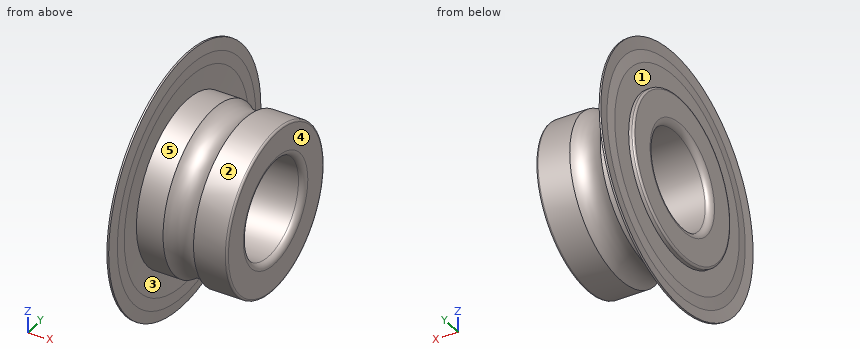
Autodesk Inventor part; units mm, degrees
ref_plane "YZ Plane" through (0, 0, 0) normal (1, 0, 0) x (0, 1, 0)
ref_plane "XZ Plane" through (0, 0, 0) normal (0, 1, 0) x (-1, 0, 0)
ref_plane "XY Plane" through (0, 0, 0) normal (0, 0, 1) x (1, 0, 0)
sketch "Sketch_62" plane through (0, 0, 0) normal (0, 0, 1) x (1, 0, 0)
  line L0 (50, 0) -> (-50, 0)
  line L1 (0, 4.1) -> (0, 2.8)
  arc A0 (0, 2.8) -> (0.3, 2.5) centre (0.3, 2.8) ccw
  line L2 (0.3, 2.5) -> (4.7, 2.5)
  arc A1 (4.7, 2.5) -> (5, 2.8) centre (4.7, 2.8) ccw
  line L3 (5, 2.8) -> (5, 4.1)
  arc A2 (5, 4.1) -> (4.9, 4.2) centre (4.9, 4.1) ccw
  line L4 (4.9, 4.2) -> (3.2793, 4.2)
  arc A3 (1.7207, 4.2) -> (3.2793, 4.2) centre (2.5, 5.1) ccw
  line L5 (1.7207, 4.2) -> (0.1, 4.2)
  arc A4 (0.1, 4.2) -> (0, 4.1) centre (0.1, 4.1) ccw
revolve "Revolution1" add sketch "Sketch_62" angle 360 about axis through (50, 0, 0) along (1, 0, 0)
sketch "Sketch_63" plane through (0, 0, 0) normal (0, 0, 1) x (1, 0, 0)
  line L0 (50, 0) -> (-50, 0)
  line L1 (0.27, 6.61) -> (0.315, 6.0075)
  line L2 (0.315, 6.0075) -> (0.27, 5.405)
  line L3 (0.27, 5.405) -> (0.27, 4.2)
  line L4 (0.27, 4.2) -> (0.36, 4.2)
  line L5 (0.36, 4.2) -> (0.45, 5.405)
  line L6 (0.45, 5.405) -> (0.45, 6.0075)
  line L7 (0.45, 6.0075) -> (0.36, 6.61)
  line L8 (0.36, 6.61) -> (0.27, 6.61)
revolve "Revolution2" add sketch "Sketch_63" angle 360 about axis through (50, 0, 0) along (1, 0, 0)
properties part number "625-Z_PART1"
For this review, take the finished solid that the model builds, in its own axes (mm). Face numbers are marked on the shaded views. A direction names the side the tool comes from. Round coordinates to 2 decimals unless told otherwise and drop trailing zeros. Loops run counter-clockwise (first coordinate to the right, second up) from the corner with the lowest first, then second, coordinate; pieces in that order, holes last. Notation, with made-up numbers: (-36.75, 46.5) - (20.25, 46.5) arc R14 cw to (20.25, 64.5) - close; hole circle Ø6 at (45, 21.5). An arc over 180 degrees is marked (long way). Put each result on its own line as item: value. Start each with the question number.
1. Mouldability with a two-part tool opening along Y and no side actions: class the marked faces 1, 2 and 3 as +Y half, -Y half, draft (parallel to the pull), parting line (faces both ways), or undercut.
2. For probe 1 along Z at (x, y) = (1.7, 0); probe 2 along Y at (x, z) = (3.6, 0.5); probe 3 along Z at (x, y) = (1.8, 0), list the stretches that pass through material, from the lowest coordinate up. Write a range as [from, to].
3. Consider section A-A on x = 4.5. State the section outline as (y, z) points.
4. For the marked faces 4 and 5, list the 3-axis set-ups (+Z, -Z, +X, -X, +Y, -Y) from which the entire face can be reached by the end or side of a thin tool; tool diameter is ignored.
5. Consider section B-B on x = 2.75. State the section outline as (y, z) points.
6. Insertion check: P1, Ø4, axis at y = -0.5, z = -0.5, coming from the -X side; P2, Ø2, axis at x = 3.5, z = -0.5, coming from the +Y side; P3, Ø1, axis at x = 1, z = 2, coming from the +Y side. Each pin has a flat end and moves straight along its axis. Give the tip position at first contact, or say it passes through.
Result sheet:
1. face 1: draft
1. face 2: parting line
1. face 3: undercut
2. probe 1: [-4.2, -2.5], [2.5, 4.2]
2. probe 2: [-4.17, -2.45], [2.45, 4.17]
2. probe 3: [-4.14, -2.5], [2.5, 4.14]
3. outline: circle Ø8.4 at (0, 0); hole circle Ø5 at (0, 0)
4. face 4: +Z, -Z, +X, +Y, -Y
4. face 5: +X
5. outline: circle Ø7.87 at (0, 0); hole circle Ø5 at (0, 0)
6. P1: x = 0.01
6. P2: y = 4.2
6. P3: y = 3.92
